For this review, take the finished solid that the model builds, in its own axes (mm). A direction names the side the tool comes from. Coordinates: 2 decimals unless noted, no trailing zeros. Write each loop counter-clockwise with the first axis right and the second up, starting at its lowest first coordinate (ties: lowest second). Pieces come first, ordered by that corner, then holes. Notation, with made-up numbers: (43.5, -33) - (76.5, -33) arc R36 cw to (76.5, 2) - close; hole circle Ø11 at (60.5, 19.5). An arc over 180 degrees is marked (long way). Use one line per item in the form item = value. Start each with the question number.
1) We need section B-B (x = 1.3). Count the separate pieces of the cut face and the enclosed holes in it, plus the area to 3 significant figures.
2) We need section C-C (y = 29.5). Give the boundary of the cut face in (x, z).
3) For L1, parallel to Y at x = 2.4, z = 12.5; L2, parallel to Z at x = 0.55, y = -11.5; L3, parallel to Z at x = 0.5, y = -9.5, list the stretches that pass through material, from the lowest coordinate up. Write a range as from..to.
4) Tool access review of faces 5 (the cylindrical face through (1.3, 21.1, 18.5)), 6 (the cylindrical face through (1.25, 33.01, 20.42)): name each direction out of +Z, -Z, +X, -X, +Y, -Y from which nothing blocks a thin tool from reaching the whole face with its end or side.
5) Mouldability with a two-part tool opening along Y and no side actions: class faces 1 (the flat face through (1.25, -25.2, -0.84)), 2 (the flat face through (2.54, 0, 2)), 3 (the flat face through (1.252, 24.953, -1.215)), 4 (the cylindrical face through (1.252, 5.691, 13.415)) as pulls with the +Y half, pulls with the -Y half, needs draft (parallel to the pull), parting line crosses it, or undercut.
6) We need section A-A (y = 0). Give the boundary of the cut face in (x, z), plus the area to 3 significant figures.
7) We need section D-D (z = -16.5). Give the boundary of the cut face in (x, y), plus the area to 3 significant figures.
8) Insertion check: P1, Ø1.5, axis at x = 0.5, y = 10.5, coming from the -Z side. The pin has a flat end and moves straight along its axis. Give the tip position at first contact, or say it passes through.
```python
from build123d import *

# Parameters (mm, degrees)
BOSS_EXTRUDE1_DEPTH   = 2.54
F_8_CLEARANCE_HOLE1_D = 4.4958
F_6_CLEARANCE_HOLE1_D = 3.7973


with BuildPart() as part:
    # Sketch1 → Boss-Extrude1 (new body)
    with BuildSketch(Plane(origin=(0, 0, 0), x_dir=(0, 0, -1), z_dir=(1, 0, 0))):
        with BuildLine():
            Line((29.249678303, 5.059653892), (14.797078303, 16.019753892))
            ThreePointArc((14.797078303, 16.019753892), (14.622989145, 16.14717462), (14.444672021, 16.268608061))
            Line((14.444672021, 16.268608061), (-12.390427979, 33.883508061))
            ThreePointArc((-12.390427979, 33.883508061), (-20.503514332, 32.92233885), (-20.955, 24.765))
            ThreePointArc((-20.955, 24.765), (-18.474577219, 21.05577373), (-16.409060049, 17.100461415))
            ThreePointArc((-16.409060049, 17.100461415), (-15.641722595, 14.450337743), (-15.666107705, 11.691467029))
            ThreePointArc((-15.666107705, 11.691467029), (-15.575146808, 9.784196429), (-14.742333624, 8.065948127))
            ThreePointArc((-14.742333624, 8.065948127), (-13.400723388, 5.655129962), (-12.806341132, 2.960937694))
            ThreePointArc((-12.806341132, 2.960937694), (-12.7, 0), (-12.806341132, -2.960937694))
            ThreePointArc((-12.806341132, -2.960937694), (-13.400723388, -5.655129962), (-14.742333624, -8.065948127))
            ThreePointArc((-14.742333624, -8.065948127), (-15.575146808, -9.784196429), (-15.666107705, -11.691467029))
            ThreePointArc((-15.666107705, -11.691467029), (-15.641722595, -14.450337743), (-16.409060049, -17.100461415))
            ThreePointArc((-16.409060049, -17.100461415), (-18.474577219, -21.05577373), (-20.955, -24.765))
            ThreePointArc((-20.955, -24.765), (-20.503514332, -32.92233885), (-12.390427979, -33.883508061))
            Line((-12.390427979, -33.883508061), (14.444672021, -16.268608061))
            ThreePointArc((14.444672021, -16.268608061), (14.622989145, -16.14717462), (14.797078303, -16.019753892))
            Line((14.797078303, -16.019753892), (29.249678303, -5.059653892))
            ThreePointArc((29.249678303, -5.059653892), (31.7627, 0), (29.249678303, 5.059653892))
        make_face()
    extrude(amount=BOSS_EXTRUDE1_DEPTH)

    # #8 Clearance Hole1 (through all)
    with Locations(Plane(origin=(2.54, 0, 0), x_dir=(0, 0, -1), z_dir=(1, 0, 0))):
        with Locations((-15.875, 28.575), (25.4127, 0), (-15.875, -28.575)):
            Hole(F_8_CLEARANCE_HOLE1_D / 2)

    # #6 Clearance Hole1 (through all)
    with Locations(Plane(origin=(2.54, 0, 0), x_dir=(0, 0, -1), z_dir=(1, 0, 0))):
        with Locations((-10.9601, 10.9601), (10.9601, 10.9601), (-10.9601, -10.9601), (10.9601, -10.9601)):
            Hole(F_6_CLEARANCE_HOLE1_D / 2)


solid = part.part
```
Determined:
q1.separate_pieces = 1
q1.enclosed_holes = 7
q1.area = 1,930 mm²
q2.outline = (0, 5.71) - (2.54, 5.71) - (2.54, 13.83) - (0, 13.83) - close; (0, 17.92) - (2.54, 17.92) - (2.54, 22.16) - (0, 22.16) - close
q3.L1 = -33.95..-12.07, -9.85..9.85, 12.07..33.95
q3.L2 = -20.76..-12.78, -9.14..9.14, 12.78..15.69
q3.L3 = -23.39..-12.17, -9.75..9.75, 12.17..15.49
q4.face_5 = +Z, +X, -X
q4.face_6 = +X, -X
q5.face_1 = pulls with the -Y half
q5.face_2 = needs draft
q5.face_3 = pulls with the +Y half
q5.face_4 = undercut
q6.outline = (0, -31.76) - (2.54, -31.76) - (2.54, -27.66) - (0, -27.66) - close; (0, -23.16) - (2.54, -23.16) - (2.54, 12.7) - (0, 12.7) - close
q6.area = 102 mm²
q7.outline = (0, -14.73) - (2.54, -14.73) - (2.54, 14.73) - (0, 14.73) - close
q7.area = 74.8 mm²
q8.P1 = -23.06
